For this review, use the dimensioned drawing (mm, ordinates from the lowest corner) and the shaded views. A direction names the side the tool comes from. Round coordinates to 2 decimals unless told otherwise and drop trailing zeros. Loops run counter-clockwise (first coordinate to the right, second up) from the corner with the lowest first, then second, coordinate; pieces in that order, holes last. Notation, with made-up numbers: M 55.25,27 L 108.25,27 A35 ccw 108.25,65 Z; hole C -1.5,77 d2. An arc over 180 degrees is marked long. Answer as a JSON object with one key per item and string values. Group by question number.
Item 1: Consider section B-B (y = 62). Give the boundary of the cut face in (x, z).
Item 2: Consider section A-A (x = 35). Give the boundary of the cut face in (y, z), and give its area (3 significant figures).
Item 3: Tool access review of the marked faces 4, 5, 6 and 7: name each direction out of +Z, -Z, +X, -X, +Y, -Y from which nothing blocks a thin tool from reaching the whole face with its end or side.
Item 4: To check wall thickness, follow line 1 (X direction, y = 49.5, z = 28) (1 decimal); line 2 (Y direction, x = 48, z = 2.5); line 3 (X direction, y = 66, z = 2.5). State the ranges of each line that lie inside material, in increasing order.
Item 5: Consider section C-C (z = 35). Give the boundary of the cut face in (x, y), and give its area (3 significant figures).
Item 6: Consider section D-D (x = 7.5). Give the boundary of the cut face in (y, z), and give its area (3 significant figures).
Item 7: The part is to be moulded in two halves that separate along Y. For the marked faces 1, 2 and 3, say which applies: +Y half, -Y half, draft (parallel to the pull), parting line (faces both ways), or undercut.
Item 8: Insertion check: P1, Ø1.5, axis at x = 28, y = 10.5, coming from the +Z side; P2, Ø5, axis at x = 15.5, z = 7.5, coming from the -Y side; P3, Ø12, axis at x = 33.5, y = 50, coming from the -Z side; P4, Ø21.5, axis at y = 14, z = 25.5, coming from the -X side. Each pin has a flat end and moves straight along its axis. Give the tip position at first contact, or say it passes through.
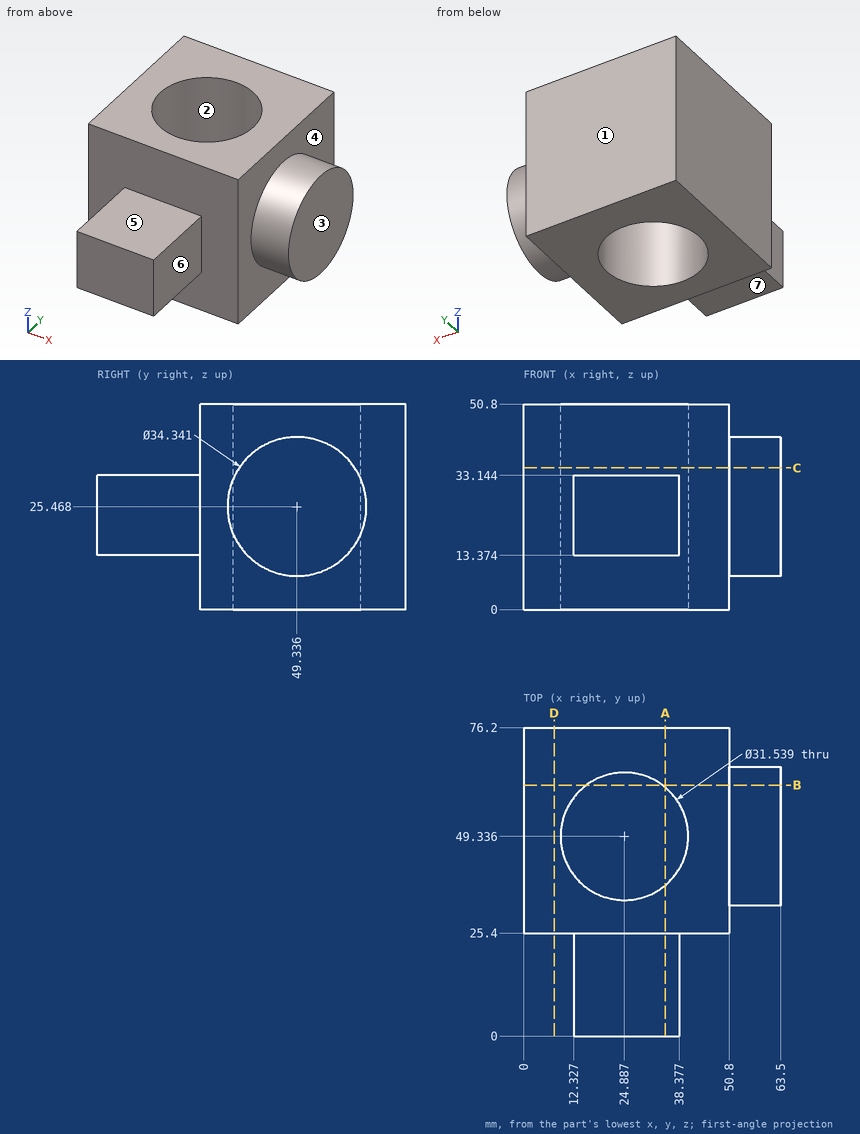
Geometry results:
{
 "1": {"outline": "M 0,0 L 15.49,0 L 15.49,50.8 L 0,50.8 Z; M 34.28,0 L 50.8,0 L 50.8,13.87 L 63.5,13.87 L 63.5,37.06 L 50.8,37.06 L 50.8,50.8 L 34.28,50.8 Z"},
 "2": {"outline": "M 0,13.37 L 25.4,13.37 L 25.4,0 L 37.24,0 L 37.24,50.8 L 25.4,50.8 L 25.4,33.14 L 0,33.14 Z; M 61.44,0 L 76.2,0 L 76.2,50.8 L 61.44,50.8 Z", "area": "1,850 mm^2"},
 "3": {"face 4": "+X", "face 5": "+Z, +X, -X, -Y", "face 6": "+Z, -Z, +X, -Y", "face 7": "-Z, +X, -X, -Y"},
 "4": {"line 1": "x = 0 to 9.1, 40.7 to 63.5", "line 2": "y = 25.4 to 76.2", "line 3": "x = 0 to 50.8"},
 "5": {"outline": "M 0,25.4 L 50.8,25.4 L 50.8,35.05 L 63.5,35.05 L 63.5,63.62 L 50.8,63.62 L 50.8,76.2 L 0,76.2 Z; hole C 24.89,49.34 d31.54", "area": "2,160 mm^2"},
 "6": {"outline": "M 25.4,0 L 76.2,0 L 76.2,50.8 L 25.4,50.8 Z", "area": "2,580 mm^2"},
 "7": {"face 1": "+Y half", "face 2": "undercut", "face 3": "draft"},
 "8": {"P1": "stops at z = 33.14", "P2": "stops at y = 25.4", "P3": "passes through", "P4": "stops at x = 12.33"}
}
